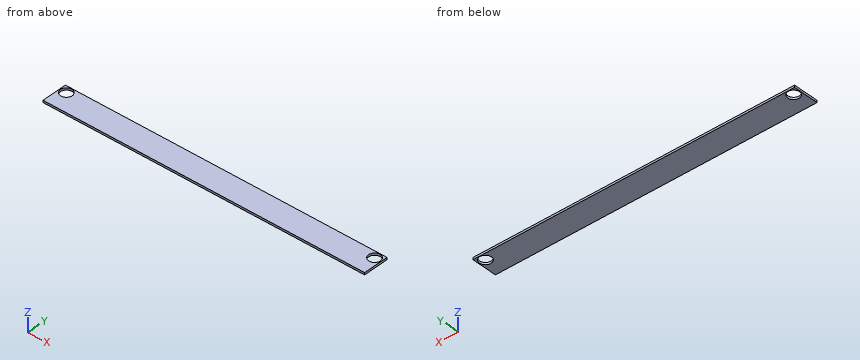
from build123d import *

# Parameters (mm, degrees)
CROQUIS1_W              = 600
CROQUIS1_H              = 47
SALIENTE_EXTRUIR1_DEPTH = 4
CROQUIS2_R              = 11
CORTAR_EXTRUIR1_DEPTH   = 4


with BuildPart() as part:
    # Croquis1 → Saliente-Extruir1 (new body)
    with BuildSketch(Plane.XY):
        with Locations((0, -11.5)):
            Rectangle(CROQUIS1_W, CROQUIS1_H)
    extrude(amount=SALIENTE_EXTRUIR1_DEPTH)

    # Croquis2 → Cortar-Extruir1 (cut)
    with BuildSketch(Plane.XY.offset(4)):
        with Locations((287.5, 0)):
            Circle(CROQUIS2_R)
        with Locations(Location((-287.5, 0, 0), (0, 0, 180))):
            Circle(CROQUIS2_R)
    extrude(amount=-CORTAR_EXTRUIR1_DEPTH, mode=Mode.SUBTRACT)


solid = part.part
Work out the finished part from the listing and answer in its coordinate system (mm). Coordinates: 2 decimals unless noted, no trailing zeros. Order: outer loops, then holes, each group sorted by start corner. A loop starts at its lowest first (then second) coordinate and runs counter-clockwise, first axis right, second up. Notation, with made-up numbers: (84, 44.25) - (119, 44.25) arc R24 ccw to (119, 80.25) - close; hole circle Ø11 at (57.25, 68.25). An arc over 180 degrees is marked (long way). Put each result on its own line as item: value. Start each with the question number.
1) Find section C-C (z = 0.75). Give the vertices of the cut face in (x, y), plus the area to 3 significant figures.
2) Find section B-B (x = 287.5). Give the vertices of the cut face in (y, z), plus the area to 3 significant figures.
3) Find section A-A (y = 0). Give the vertices of the cut face in (x, z).
4) Find the intervals of material crossed by line 1 (X direction, y = 1.5, z = 1.15); line 2 (Y direction, x = 287.5, z = 1.25); line 3 (X direction, y = -8, z = 1.35), in increasing order. Write a range as from..to.
Results list:
1. outline: (-300, -35) - (300, -35) - (300, 12) - (-300, 12) - close; hole circle Ø22 at (-287.5, 0); hole circle Ø22 at (287.5, 0)
1. area: 27,400 mm^2
2. outline: (-35, 0) - (-11, 0) - (-11, 4) - (-35, 4) - close; (11, 0) - (12, 0) - (12, 4) - (11, 4) - close
2. area: 100 mm^2
3. outline: (-300, 0) - (-298.5, 0) - (-298.5, 4) - (-300, 4) - close; (-276.5, 0) - (276.5, 0) - (276.5, 4) - (-276.5, 4) - close; (298.5, 0) - (300, 0) - (300, 4) - (298.5, 4) - close
4. line 1: x = -300..-298.4, -276.6..276.6, 298.4..300
4. line 2: y = -35..-11, 11..12
4. line 3: x = -300..-295.05, -279.95..279.95, 295.05..300
